```python
from build123d import *

# Parameters (mm, degrees)
CUT_EXTRUDE7_DEPTH      = 57.29387178
CUT_EXTRUDE7_DEPTH_BACK = 57.29387178
SKETCH7_R               = 10
CHAMFER6_SIZE           = 0.25
CHAMFER7_SIZE           = 0.25


with BuildPart() as part:
    # Sketch1 → Revolve4 (revolve)
    with BuildSketch(Plane(origin=(0, 0, 0), x_dir=(0, 0, -1), z_dir=(1, 0, 0)), mode=Mode.PRIVATE) as revolve4_sk:
        with BuildLine():
            Line((30, 37), (0, 37))
            Line((0, 37), (0, 25))
            Line((0, 25), (22, 25))
            ThreePointArc((22, 25), (23.414213562, 24.414213562), (24, 23))
            Line((24, 23), (24, 15))
            ThreePointArc((24, 15), (23.414213562, 13.585786438), (22, 13))
            Line((22, 13), (10, 13))
            Line((10, 13), (10, -13))
            Line((10, -13), (27, -13))
            Line((27, -13), (27, -32))
            Line((27, -32), (0, -32))
            Line((0, -32), (0, -35))
            Line((0, -35), (30, -35))
            Line((30, -35), (30, 13))
            Line((30, 13), (27, 13))
            Line((27, 13), (27, 16))
            Line((27, 16), (30, 16))
            Line((30, 16), (30, 19))
            Line((30, 19), (27, 19))
            Line((27, 19), (27, 22))
            Line((27, 22), (30, 22))
            Line((30, 22), (30, 25))
            Line((30, 25), (27, 25))
            Line((27, 25), (27, 28))
            Line((27, 28), (30, 28))
            Line((30, 28), (30, 31))
            Line((30, 31), (27, 31))
            Line((27, 31), (27, 34))
            Line((27, 34), (30, 34))
            Line((30, 34), (30, 37))
        make_face()
    revolve(revolve4_sk.sketch.rotate(Axis((0, 50, 0), (0, -1, 0)), 180), axis=Axis((0, 50, 0), (0, -1, 0)))

    # Sketch7 → Cut-Extrude7 (cut, two sides: drawn at the far end of the back side and taken through both)
    with BuildSketch(Plane.XY.offset(-CUT_EXTRUDE7_DEPTH_BACK)):
        Circle(SKETCH7_R)
    extrude(amount=CUT_EXTRUDE7_DEPTH + CUT_EXTRUDE7_DEPTH_BACK, mode=Mode.SUBTRACT)

    # Chamfer6
    chamfer6_edges = [part.edges().sort_by_distance(p)[0] for p in [
        (0, -32, -27),
    ]]
    chamfer(chamfer6_edges, length=CHAMFER6_SIZE)

    # Chamfer7
    chamfer7_edges = [part.edges().sort_by_distance(p)[0] for p in [
        (0, -13, -27),
    ]]
    chamfer(chamfer7_edges, length=CHAMFER7_SIZE)


solid = part.part
```
Source: CAD feature listing. Evaluate the final solid. Frame: model axes, mm. A direction names the side the tool comes from. Coordinates: 2 decimals unless noted, no trailing zeros. Loops run counter-clockwise (first coordinate to the right, second up) from the corner with the lowest first, then second, coordinate; pieces in that order, holes last. Notation, with made-up numbers: (34, 2) - (47, 2) arc R12 ccw to (47, 22) - close; hole circle Ø1 at (-9, 11). An arc over 180 degrees is marked (long way). Answer as CSV lines item,"result".
1. Contact query for flat-ended pins moving along their axis: pin 1 (5 mm diameter, centred on y = 27, z = 9.5, fed in from -X); pin 2 (1.5 mm diameter, centred on y = -23, z = 6.5, fed in from +X); pin 3 (8 mm diameter, centred on y = -13, z = -4.5, fed in from +X). Output: stop coordinate, or through.
Established:
pin 1,"stops at x = -29.12"
pin 2,"stops at x = 29.44"
pin 3,"stops at x = 30"
2. Ray query, line 1 (Y direction, x = 19.5, z = -5); line 2 (Y direction, x = 20.5, z = 19); line 3 (Y direction, x = -3, z = -14.5). Return the intervals inside material, ascending.
Established:
line 1,"y = -35 to -32, -13 to 13, 25 to 37"
line 2,"y = -35 to 13, 16 to 19, 22 to 25, 28 to 31, 34 to 37"
line 3,"y = -35 to -32, -13 to -9.54, 9.54 to 13, 25 to 37"
3. Section B-B (y = -1). Return loops of the section in (x, z), then the cut area to 3 significant figures.
Established:
outline,"(-9.95, -28.3) - (-9.95, -1) arc R10 cw to (-9.95, 1) - (-9.95, 28.3) arc R30 ccw to start; (9.95, -28.3) arc R30 ccw to (9.95, 28.3) - (9.95, 1) arc R10 cw to (9.95, -1) - close"
area,"1,660 mm2"
4. Section A-A (y = -8.5). Return loops of the section in (x, z), then the cut area to 3 significant figures.
Established:
outline,"(-5.27, -29.53) - (-5.27, -8.5) arc R10 cw to (-5.27, 8.5) - (-5.27, 29.53) arc R30 ccw to start; (5.27, -29.53) arc R30 ccw to (5.27, 29.53) - (5.27, 8.5) arc R10 cw to (5.27, -8.5) - close"
area,"2,080 mm2"
5. Mould query, pull axis X, two halves, no side actions, for faces 3 (the flat face through (-11, 34, 25)), 4 (the cylindrical face through (-7.21, 18.94, 22.89)), 5 (the cylindrical face through (-25.296, 35.521, 16.128)). Classes: released by +X, released by -X, zero draft, split by the parting line, or undercut.
Established:
face 3,"zero draft"
face 4,"undercut"
face 5,"split by the parting line"
6. Reachability of faces 1 (the cylindrical face through (11.49, -10.664, 27.712)), 2 (the flat face through (12, -13, 0)) from +Z, -Z, +X, -X, +Y, -Y: full face, straight path, thin tool, end or side. Return the list, or none.
Established:
face 1,"+Y, -Y"
face 2,"none"
7. Section C-C (z = 18.5). Count the separate pieces of the cut face and the enclosed holes in it, then the cut area to 3 significant figures.
Established:
separate pieces,"1"
enclosed holes,"3"
area,"1,880 mm2"
